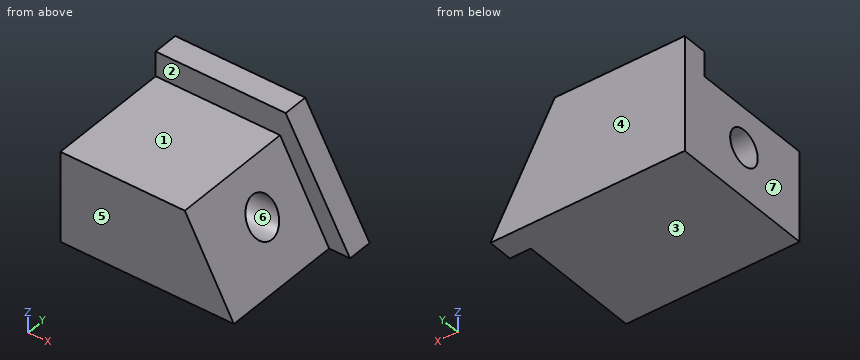
```python
from build123d import *

# Parameters (mm, degrees)
F0_W     = 107.3800772429
F0_H     = 82.039296627
F1_DEPTH = 63.5
F3_DEPTH = 82.040296627
F5_DEPTH = 68.072
F6_R     = 9.8390398468
F7_DEPTH = 107.3810772429


with BuildPart() as f1:
    # F0 (on Top) → F1 (new body)
    with BuildSketch(Plane.XY):
        with Locations((-0.9704492986, 1.2810640037)):
            Rectangle(F0_W, F0_H)
    extrude(amount=F1_DEPTH)

    # F2 (on face) → F3 (cut, through all)
    with BuildSketch(Plane.XZ.offset(39.7385843098)):
        Polygon((17.1634294093, 63.5), (52.7195893228, 0), (52.7195893228, 63.5), align=None)
    extrude(amount=-F3_DEPTH, mode=Mode.SUBTRACT)

    # F4 (on face) → F5 (cut)
    with BuildSketch(Plane.XZ.offset(39.7385843098)):
        Polygon((17.1634294093, 63.5), (-54.66048792, 63.5), (-54.66048792, 49.8112104833), (14.0662752092, 49.8112104833), (41.1664322019, 0), (52.7195893228, 0), align=None)
    extrude(amount=-F5_DEPTH, mode=Mode.SUBTRACT)

    # F6 (on face) → F7 (cut, through all)
    with BuildSketch(Plane(origin=(-54.66048792, 0, 0), x_dir=(0, -1, 0), z_dir=(-1, 0, 0))):
        with Locations((0, 27.6148878038)):
            Circle(F6_R)
    extrude(amount=-F7_DEPTH, mode=Mode.SUBTRACT)


solid = f1.part
```
Check sheet for the modelled part. Datum: model origin and axes. Units: mm. Face numbers are marked on the shaded views. A direction names the side the tool comes from. Give positions to 0.01 mm unless a question says otherwise; leave off trailing zeros. Order: outer loops, then holes, each group sorted by start corner. A loop starts at its lowest first (then second) coordinate and runs counter-clockwise, first axis right, second up. Notation, with made-up numbers: M 80.5,71 L 89.5,71 A20 ccw 89.5,97 Z; hole C 25.5,44.25 d4. An arc over 180 degrees is marked long. Answer in a Markdown table with one row per item. Add a question column.
Q1. Access from +Z, -Z, +X, -X, +Y, -Y to the whole of each face (thin tool, end or side, straight path). Record for the marked faces 1, 2 and 3.
Q2. Thickness scan on L1, parallel to Z at x = -18, y = 0; L2, parallel to Z at x = -34, y = -29; L3, parallel to Y at x = -47, z = 57. Record the ranges inside material, lowest first.
Q3. Sectioned sample at A-A, the plane z = 35.5. Record the boundary of the cut face in (x, y), and give its area (3 significant figures).
Q4. Gauge pin test, flat ends, axial feed: pin 1 Ø2 at (y, z) = (-13.5, 8.5) entering from +X; pin 2 Ø15.5 at (y, z) = (0, 27.61) entering from -X; pin 3 Ø3 at (x, y) = (25, -31) entering from +Z; pin 4 Ø8 at (x, y) = (1, 15) entering from +Z. Record the tip position at first contact, or that the pin passes through.
Q5. Release check for a two-part mould opening along Y. For the marked faces 4, 5, 6 and 7 record: released by +Y, released by -Y, zero draft, split by the parting line, or undercut.
Q6. Sectioned sample at B-B, the plane y = -4. Record the boundary of the cut face in (x, z).
Q7. Sectioned sample at C-C, the plane x = 23. Record the boundary of the cut face in (y, z).
Q8. Sectioned sample at D-D, the plane x = 4. Record the boundary of the cut face in (y, z), and give its area (3 significant figures).
Verdict:
| question | item | result |
|---|---|---|
| 1 | face 1 | +Z, +X, -X, -Y |
| 1 | face 2 | +Z, +X, -Y |
| 1 | face 3 | -Z, +X, -X, +Y, -Y |
| 2 | L1 | 0 to 17.78, 37.45 to 49.81 |
| 2 | L2 | 0 to 49.81 |
| 2 | L3 | 28.33 to 42.3 |
| 3 | outline | M -54.66,-39.74 L 21.85,-39.74 L 21.85,-5.88 L -54.66,-5.88 Z; M -54.66,5.88 L 21.85,5.88 L 21.85,28.33 L 32.84,28.33 L 32.84,42.3 L -54.66,42.3 Z |
| 3 | area | 5,530 mm² |
| 4 | pin 1 | x = 37.09 |
| 4 | pin 2 | through |
| 4 | pin 3 | z = 32.47 |
| 4 | pin 4 | z = 49.81 |
| 5 | face 4 | released by +Y |
| 5 | face 5 | released by -Y |
| 5 | face 6 | undercut |
| 5 | face 7 | zero draft |
| 6 | outline | M -54.66,0 L 41.17,0 L 31.03,18.63 L -54.66,18.63 Z; M -54.66,36.6 L 21.25,36.6 L 14.07,49.81 L -54.66,49.81 Z |
| 7 | outline | M -39.74,0 L 42.3,0 L 42.3,53.08 L 28.33,53.08 L 28.33,33.39 L 7.97,33.39 A9.84 cw long -7.97,33.39 L -39.74,33.39 Z |
| 8 | outline | M -39.74,0 L 42.3,0 L 42.3,63.5 L 28.33,63.5 L 28.33,49.81 L -39.74,49.81 Z; hole C 0,27.61 d19.68 |
| 8 | area | 3,970 mm² |
